Part model, mm, in its own coordinate system. A direction names the side the tool comes from. Coordinates: 2 decimals unless noted, no trailing zeros. Loops run counter-clockwise (first coordinate to the right, second up) from the corner with the lowest first, then second, coordinate; pieces in that order, holes last.
```python
from build123d import *

# Parameters (mm, degrees)
BOSS_EXTRUDE1_DEPTH = 3
FILLET1_R           = 0.5
FILLET2_R           = 2
SKETCH2_R           = 1
CUT_EXTRUDE1_DEPTH  = 3


with BuildPart() as part:
    # Sketch1 → Boss-Extrude1 (new body)
    with BuildSketch(Plane.XY):
        Polygon((-3.175426481, 5.5), (3.175426481, 5.5), (6.350852961, 0), (3.175426481, -5.5), (-3.175426481, -5.5), (-3.175426481, -8.5), (36.824573519, -8.5), (36.824573519, -5), (31.051070828, -5), (28.164319482, 0), (31.051070828, 5), (36.824573519, 5), (36.824573519, 8.5), (-3.175426481, 8.5), align=None)
    extrude(amount=BOSS_EXTRUDE1_DEPTH)

    # Fillet1
    fillet1_edges = [part.edges().sort_by_distance(p)[0] for p in [
        (36.824573519, -5, 1.5),
        (-3.175426481, -5.5, 1.5),
        (-3.175426481, 5.5, 1.5),
        (36.824573519, 5, 1.5),
    ]]
    fillet(fillet1_edges, radius=FILLET1_R)

    # Fillet2
    fillet2_edges = [part.edges().sort_by_distance(p)[0] for p in [
        (36.824573519, -8.5, 1.5),
        (-3.175426481, -8.5, 1.5),
        (-3.175426481, 8.5, 1.5),
        (36.824573519, 8.5, 1.5),
    ]]
    fillet(fillet2_edges, radius=FILLET2_R)

    # Sketch2 → Cut-Extrude1 (cut)
    with BuildSketch(Plane.XY.offset(3)):
        with Locations((9.526279442, 4.5)):
            Circle(SKETCH2_R)
    extrude(amount=-CUT_EXTRUDE1_DEPTH, mode=Mode.SUBTRACT)


solid = part.part
```
Q1. Saw through at B-B (y = 4.5). List the corners of the cut face in (x, z), plus the area to 3 significant figures.
Q2. Tool access for faces 1 (the flat face through (29.628, -2.535, 1.479)), 2 (the flat face through (0, -5.5, 1)), 3 (the flat face through (17, -8.5, 1)): list every direction of +Z, -Z, +X, -X, +Y, -Y with a clear straight run to the whole face (end or side of a thin tool).
Q3. Mould opens along Y. For faces 4 (the flat face through (0, 5.5, 1)), 5 (the cylindrical face through (36.22, -7.93, 1.52)), 6 (the flat face through (17, 8.5, 1)) say: released by +Y, released by -Y, zero draft, split by the parting line, or undercut.
Q4. Saw through at D-D (y = 1.5). List the corners of the cut face in (x, z).
Q5. Saw through at C-C (z = 1.1). List the corners of the cut face in (x, y), plus the area to 3 significant figures.
Q6. Saw through at A-A (x = 0.5). List the corners of the cut face in (y, z).
Q7. Probe line 1 (Y direction, x = 33, z = 2.15); line 2 (Y direction, x = 0.5, z = 2.5); line 3 (X direction, y = 3.75, z = 1.2). List the from-to ranges inside material, lowest first.
Checked values:
1. outline: (3.75, 0) - (8.53, 0) - (8.53, 3) - (3.75, 3) - close; (10.53, 0) - (30.76, 0) - (30.76, 3) - (10.53, 3) - close
1. area: 75.0 mm2
2. face 1: +Z, -Z, +X
2. face 2: +Z, -Z, -X
2. face 3: +Z, -Z, +X, -X, -Y
3. face 4: undercut
3. face 5: released by -Y
3. face 6: released by +Y
4. outline: (5.48, 0) - (29.03, 0) - (29.03, 3) - (5.48, 3) - close
5. outline: (-3.18, -6.5) arc R2 ccw to (-1.18, -8.5) - (34.82, -8.5) arc R2 ccw to (36.82, -6.5) - (36.82, -5.5) arc R0.5 ccw to (36.32, -5) - (31.05, -5) - (28.16, 0) - (31.05, 5) - (36.32, 5) arc R0.5 ccw to (36.82, 5.5) - (36.82, 6.5) arc R2 ccw to (34.82, 8.5) - (-1.18, 8.5) arc R2 ccw to (-3.18, 6.5) - (-3.18, 6) arc R0.5 ccw to (-2.68, 5.5) - (3.18, 5.5) - (6.35, 0) - (3.18, -5.5) - (-2.68, -5.5) arc R0.5 ccw to (-3.18, -6) - close; hole circle Ø2 at (9.53, 4.5)
5. area: 514 mm2
6. outline: (-8.5, 0) - (-5.5, 0) - (-5.5, 3) - (-8.5, 3) - close; (5.5, 0) - (8.5, 0) - (8.5, 3) - (5.5, 3) - close
7. line 1: y = -8.5 to -5, 5 to 8.5
7. line 2: y = -8.5 to -5.5, 5.5 to 8.5
7. line 3: x = 4.19 to 8.86, 10.19 to 30.33
